Print and shaded views of the part. All mm, measured from the part's lowest x, y and z. A direction names the side the tool comes from. Round coordinates to 2 decimals unless told otherwise and drop trailing zeros. Order: outer loops, then holes, each group sorted by start corner. A loop starts at its lowest first (then second) coordinate and runs counter-clockwise, first axis right, second up. Notation, with made-up numbers: (-39.5, -17) - (-28.5, -17) arc R15 cw to (-28.5, -4) - close; hole circle Ø7 at (28.25, -12). An arc over 180 degrees is marked (long way). Write item = value, one per line. Start each with the question number.
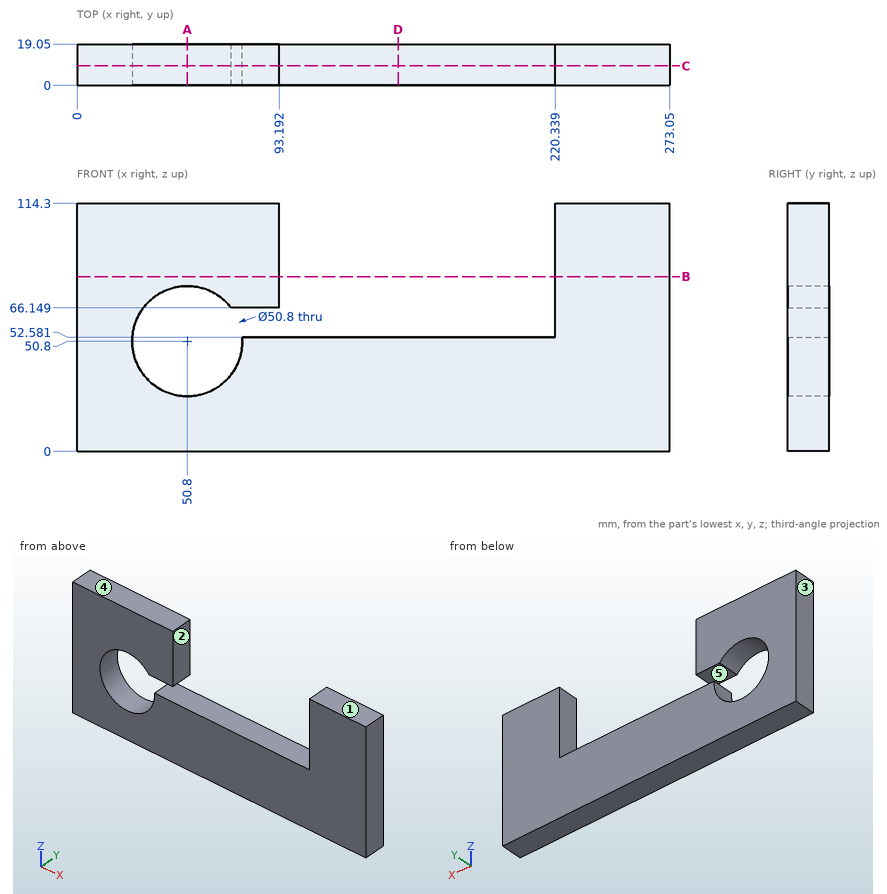
Item 1: Saw through at C-C, the plane y = 9. Give the cut face in (x, z), then the cut area to 3 significant figures.
Item 2: Saw through at D-D, the plane x = 148. Give the cut face in (y, z), then the cut area to 3 significant figures.
Item 3: Probe L1, parallel to X at y = 1.25, z = 108; L2, parallel to Z at x = 50.8, y = 15.25; L3, parallel to X at y = 6, z = 49.5. List the from-to ranges inside material, lowest first.
Item 4: Drop flat-ended pins along their axis: pin 1 (8 mm diameter, centred on x = 188.5, y = 13, fed in from +Z); pin 2 (8 mm diameter, centred on x = 99.5, z = 78.5, fed in from +Y). Give the stop position or say it passes through.
Item 5: Which spindle directions (+Z, -Z, +X, -X, +Y, -Y) get a long thin tool onto all of the face, cutting with end or side? Do the marked faces 1 and 2. Say none if no direction does.
Item 6: Saw through at A-A, the plane x = 50.8. Give the cut face in (y, z).
Item 7: Mould opens along X. For the marked faces 3, 4 and 5 say: +X half, -X half, draft (parallel to the pull), parting line (faces both ways), or undercut.
Item 8: Saw through at B-B, the plane z = 80.5. Give the cut face in (x, y), then the cut area to 3 significant figures.
Check sheet entries:
q1.outline = (0, 0) - (273.05, 0) - (273.05, 114.3) - (220.34, 114.3) - (220.34, 52.58) - (76.14, 52.58) arc R25.4 cw (long way) to (71.04, 66.15) - (93.19, 66.15) - (93.19, 114.3) - (0, 114.3) - close
q1.area = 21,100 mm2
q2.outline = (0, 0) - (19.05, 0) - (19.05, 52.58) - (0, 52.58) - close
q2.area = 1,000 mm2
q3.L1 = 0 to 93.19, 220.34 to 273.05
q3.L2 = 0 to 25.4, 76.2 to 114.3
q3.L3 = 0 to 25.43, 76.17 to 273.05
q4.pin_1 = 52.58
q4.pin_2 = through
q5.face_1 = +Z, +X, -X, +Y, -Y
q5.face_2 = +Z, +Y, -Y
q6.outline = (0, 0) - (19.05, 0) - (19.05, 25.4) - (0, 25.4) - close; (0, 76.2) - (19.05, 76.2) - (19.05, 114.3) - (0, 114.3) - close
q7.face_3 = -X half
q7.face_4 = draft
q7.face_5 = undercut
q8.outline = (0, 0) - (93.19, 0) - (93.19, 19.05) - (0, 19.05) - close; (220.34, 0) - (273.05, 0) - (273.05, 19.05) - (220.34, 19.05) - close
q8.area = 2,780 mm2
